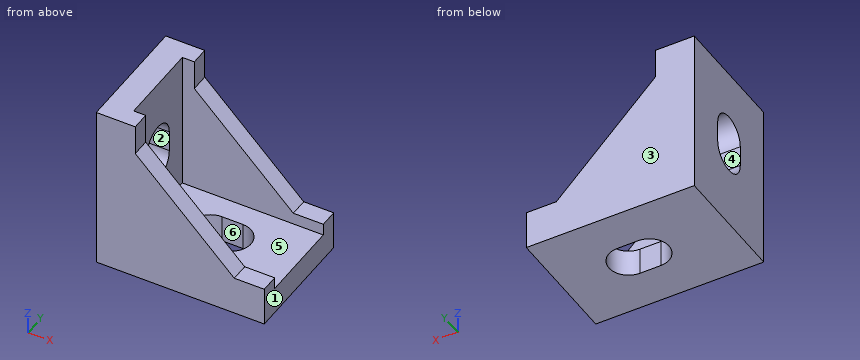
```python
from build123d import *

# Parameters (mm, degrees)
SKETCH1_W           = 28
SKETCH1_H           = 20
BOSS_EXTRUDE1_DEPTH = 4.5
CUT_EXTRUDE1_DEPTH  = 22
BOSS_EXTRUDE3_DEPTH = 3


with BuildPart() as part:
    # Sketch1 → Boss-Extrude1 (new body)
    with BuildSketch(Plane.XY):
        Rectangle(SKETCH1_W, SKETCH1_H)
        with BuildLine():
            Line((-0.75, 3.25), (2.75, 3.25))
            ThreePointArc((2.75, 3.25), (6, 0), (2.75, -3.25))
            Line((2.75, -3.25), (-0.75, -3.25))
            ThreePointArc((-0.75, -3.25), (-4, 0), (-0.75, 3.25))
        make_face(mode=Mode.SUBTRACT)
    extrude(amount=BOSS_EXTRUDE1_DEPTH)

    # Sketch3 → Cut-Extrude1 (cut)
    with BuildSketch(Plane(origin=(0, -10, 0), x_dir=(-1, 0, 0), z_dir=(0, -1, 0))):
        Polygon((14, 0), (9.5, -4.5), (14, -4.5), align=None)
    extrude(amount=-CUT_EXTRUDE1_DEPTH, mode=Mode.SUBTRACT)

    # Sketch4 → Boss-Extrude3 (add)
    with BuildSketch(Plane(origin=(0, -10, 0), x_dir=(-1, 0, 0), z_dir=(0, -1, 0))):
        Polygon((-14, -4.5), (-14, -6.5), (-9, -6.5), (-0.75, -14.75), (9.5, -4.5), align=None)
    boss_extrude3 = extrude(amount=-BOSS_EXTRUDE3_DEPTH)

    # Mirror1: Boss-Extrude3 across plane
    add(boss_extrude3.mirror(Plane(origin=(0, 0, 0), x_dir=(0, 0, 1), z_dir=(0, -1, 0))))

    # Mirror2: part across plane


with BuildPart() as part_1:
    add(part.part)
    add(part.part.mirror(Plane(origin=(-14, 12, 0), x_dir=(0.7071067811865476, 0, 0.7071067811865476), z_dir=(0.7071067811865477, 0, -0.7071067811865475))))


solid = part_1.part
```
CAD build for the part. Positions are in the model's coordinates, mm. Face numbers are marked on the shaded views. A direction names the side the tool comes from. Round coordinates to 2 decimals unless told otherwise and drop trailing zeros. Order: outer loops, then holes, each group sorted by start corner. A loop starts at its lowest first (then second) coordinate and runs counter-clockwise, first axis right, second up. Notation, with made-up numbers: (6, 63) -> (63, 63) arc R10 cw to (63, 81) -> close; hole circle Ø7 at (-27.5, -15.5). An arc over 180 degrees is marked (long way). One line per question, with ' | ' between items.
Q1. Slice it at A-A (y = 0). Write the cut outline in (x, z).
Completed:
outline: (-14, 0) -> (-4, 0) -> (-4, 4.5) -> (-9.5, 4.5) -> (-9.5, 10) -> (-14, 10) -> close; (-14, 20) -> (-9.5, 20) -> (-9.5, 28) -> (-14, 28) -> close; (6, 0) -> (14, 0) -> (14, 4.5) -> (6, 4.5) -> close
Q2. Probe probe 1 along Y at (x, z) = (-10.75, 16.5); probe 2 along Y at (x, z) = (-2.5, 9.75); probe 3 along X at (y, z) = (-4.5, 10). List the from-to ranges inside material, lowest first.
Completed:
probe 1: y = -10 to -3.25, 3.25 to 10 | probe 2: y = -10 to -7, 7 to 10 | probe 3: x = -14 to -9.5
Q3. Slice it at B-B (z = 15.25). Write the cut outline in (x, y).
Completed:
outline: (-14, -10) -> (0.25, -10) -> (0.25, -7) -> (-9.5, -7) -> (-9.5, -3.25) -> (-14, -3.25) -> close; (-14, 3.25) -> (-9.5, 3.25) -> (-9.5, 7) -> (0.25, 7) -> (0.25, 10) -> (-14, 10) -> close
Q4. Slice it at C-C (x = -10.75). Write the cut outline in (y, z).
Completed:
outline: (-10, 0) -> (10, 0) -> (10, 28) -> (-10, 28) -> close; hole (-3.25, 13.25) arc R3.25 ccw to (3.25, 13.25) -> (3.25, 16.75) arc R3.25 ccw to (-3.25, 16.75) -> close
Q5. Two-plate mould, pull along Y, no slides. Class the marked faces 1, 2 and 3: released by +Y, released by -Y, zero draft, split by the parting line, or undercut.
Completed:
face 1: zero draft | face 2: undercut | face 3: released by +Y
Q6. Which spindle directions (+Z, -Z, +X, -X, +Y, -Y) get a long thin tool onto all of the face, cutting with end or side? Do the marked faces 4, 5 and 6. Say none if no direction does.
Completed:
face 4: +X, -X | face 5: +Z, +X | face 6: +Z, -Z
Q7. Slice it at D-D (z = 9.5). Write the cut outline in (x, y), then the cut area to 3 significant figures.
Completed:
outline: (-14, -10) -> (6, -10) -> (6, -7) -> (-9.5, -7) -> (-9.5, 7) -> (6, 7) -> (6, 10) -> (-14, 10) -> close | area: 183 mm^2
Q8. Drop flat-ended pins along their axis: pin 1 (6 mm diameter, centred on x = 9.5, y = 0.5, fed in from +Z); pin 2 (1.5 mm diameter, centred on y = 3.5, z = 7.5, fed in from +X); pin 3 (0.9 mm diameter, centred on y = 9, z = 24.5, fed in from +X). Give the stop position or say it passes through.
Completed:
pin 1: stops at z = 4.5 | pin 2: stops at x = -9.5 | pin 3: stops at x = -7.5
